from build123d import *

# Parameters (mm, degrees)
BOSS_EXTRUDE1_DEPTH     = 3
SKETCH2_W               = 33
SKETCH2_H               = 10
SKETCH2_R               = 1.25
BOSS_EXTRUDE2_DEPTH     = 3
SKETCH3_R               = 1.25
CUT_EXTRUDE1_DEPTH      = 111.114926801
BOSS_EXTRUDE3_DEPTH     = 10
CUT_EXTRUDE2_REACH      = 107.286
CUT_EXTRUDE2_END_RADIUS = 197.003812576
SKETCH8_R               = 1.5
CUT_EXTRUDE3_REACH      = 97.662
CUT_EXTRUDE3_END_RADIUS = 197.003812576
SKETCH9_R               = 1.5


with BuildPart() as part:
    # Sketch1 → Boss-Extrude1 (new body)
    with BuildSketch(Plane(origin=(0, 0, 0), x_dir=(1, 0, 0), z_dir=(0, 1, 0))):
        with BuildLine():
            Line((0, 45), (0, 0))
            Line((0, 0), (7, 0))
            Line((7, 0), (45.00148551, -17.720383715))
            Line((45.00148551, -17.720383715), (43.311012463, -21.345614863))
            Line((43.311012463, -21.345614863), (100.00148551, -17.720383715))
            Line((100.00148551, -17.720383715), (100.00148551, 12.279616285))
            ThreePointArc((100.00148551, 12.279616285), (52.191052923, 35.333931061), (0, 45))
        make_face()
    extrude(amount=BOSS_EXTRUDE1_DEPTH)

    # Sketch2 → Boss-Extrude2 (add)
    with BuildSketch(Plane(origin=(1.250243366, 0, -2.681155551), x_dir=(0.9063077870366495, 0, 0.42261826174070033), z_dir=(-0.42261826174070033, 0, 0.9063077870366495))):
        with Locations((22.844154509, 5)):
            Rectangle(SKETCH2_W, SKETCH2_H)
        with Locations((13.344154509, 6)):
            Circle(SKETCH2_R, mode=Mode.SUBTRACT)
        with Locations((32.344154509, 6)):
            Circle(SKETCH2_R, mode=Mode.SUBTRACT)
    extrude(amount=-BOSS_EXTRUDE2_DEPTH)

    # Sketch3 → Cut-Extrude1 (cut, through all)
    with BuildSketch(Plane.XZ):
        with Locations(Location((5, -23.5, 0), (0, 0, 270))):
            Circle(SKETCH3_R)
        with Locations(Location((92.00148551, 2.720383715, 0), (0, 0, 270))):
            Circle(SKETCH3_R)
    extrude(amount=-CUT_EXTRUDE1_DEPTH, mode=Mode.SUBTRACT)

    # Sketch6 → Boss-Extrude3 (add)
    with BuildSketch(Plane(origin=(0, 3, 0), x_dir=(1, 0, 0), z_dir=(0, 1, 0))):
        with BuildLine():
            ThreePointArc((25.815183319, 42.016667614), (17.915864182, 43.291962745), (9.971855225, 44.250264466))
            Line((9.971855225, 44.250264466), (9.971855225, 41.238788581))
            ThreePointArc((9.971855225, 41.238788581), (17.646509134, 40.304062324), (25.278576941, 39.068923955))
            Line((25.278576941, 39.068923955), (25.815183319, 42.016667614))
        make_face()
        with BuildLine():
            ThreePointArc((91.515126037, 17.56938971), (84.541117021, 21.492248202), (77.415775106, 25.13300679))
            Line((77.415775106, 25.13300679), (76.106143507, 22.438196193))
            ThreePointArc((76.106143507, 22.438196193), (83.124741123, 18.85197958), (89.994272948, 14.987889185))
            Line((89.994272948, 14.987889185), (91.515126037, 17.56938971))
        make_face()
    extrude(amount=BOSS_EXTRUDE3_DEPTH)

    # Cut-Extrude2: up to this cylinder (the profile starts outside it)
    cut_extrude2_end = Plane(origin=(-10.004096478, 8, 154.749638432), z_dir=(0, -1, 0)) * Cylinder(CUT_EXTRUDE2_END_RADIUS, 609.579625152, mode=Mode.PRIVATE)
    # Sketch8 → Cut-Extrude2 (cut, up to the surface)
    with BuildSketch(Plane(origin=(17.915864182, 13, -43.291962745), x_dir=(-0.9902080058846244, 0, -0.13959980330213892), z_dir=(0.13959980330213892, 0, -0.9902080058846244)), mode=Mode.PRIVATE) as cut_extrude2_sk1:
        with Locations((0, -5)):
            Circle(SKETCH8_R)
    cut_extrude2_tool1 = extrude(cut_extrude2_sk1.sketch, amount=-CUT_EXTRUDE2_REACH, mode=Mode.PRIVATE) - cut_extrude2_end
    add(cut_extrude2_tool1.solids().sort_by_distance((17.915864, 8, -43.291963))[0], mode=Mode.SUBTRACT)

    # Cut-Extrude3: up to this cylinder (the profile starts outside it)
    cut_extrude3_end = Plane(origin=(-10.004096478, 8, 154.749638432), z_dir=(0, -1, 0)) * Cylinder(CUT_EXTRUDE3_END_RADIUS, 590.331625152, mode=Mode.PRIVATE)
    # Sketch9 → Cut-Extrude3 (cut, up to the surface)
    with BuildSketch(Plane(origin=(84.541117021, 13, -21.492248202), x_dir=(-0.8812094331704029, 0, -0.4727260674973377), z_dir=(0.4727260674973377, 0, -0.8812094331704029)), mode=Mode.PRIVATE) as cut_extrude3_sk1:
        with Locations((0, -5)):
            Circle(SKETCH9_R)
    cut_extrude3_tool1 = extrude(cut_extrude3_sk1.sketch, amount=-CUT_EXTRUDE3_REACH, mode=Mode.PRIVATE) - cut_extrude3_end
    add(cut_extrude3_tool1.solids().sort_by_distance((84.541117, 8, -21.492248))[0], mode=Mode.SUBTRACT)


solid = part.part
Part model, mm, in its own coordinate system. A direction names the side the tool comes from. Coordinates: 2 decimals unless noted, no trailing zeros. Loops run counter-clockwise (first coordinate to the right, second up) from the corner with the lowest first, then second, coordinate; pieces in that order, holes last. Notation, with made-up numbers: (-6.75, 31) - (14.25, 31) arc R37 ccw to (14.25, 69) - close; hole circle Ø7 at (17.5, 65). An arc over 180 degrees is marked (long way). Write each question's results on one line, items separated by ' | '. Start each with the question number.
Q1. Which spindle directions (+Z, -Z, +X, -X, +Y, -Y) get a long thin tool onto all of the face, cutting with end or side? Do faces 5 (the flat face through (22, 10, 6)), 6 (the cylindrical face through (19.24, 7.93, -40.07)), 7 (the flat face through (7.625, 6.451, -1.34)), 8 (the flat face through (90.744, 7.93, -16.261)), 9 (the cylindrical face through (81.48, 7.93, -19.724)). Say none if no direction does.
Q2. Two-plate mould, pull along Y, no slides. Class faces 1 (the cylindrical face through (13.72, 4.78, 1.5)), 2 (the flat face through (0, 1, -23)), 3 (the flat face through (49, 0, -12)), 4 (the flat face through (84, 13, -20)): +Y half, -Y half, draft (parallel to the pull), parting line (faces both ways), or undercut.
Q3. Slice it at B-B on x = 5. Give the cut face in (y, z), and give its area (3 significant figures).
Q4. Slice it at A-A on z = -23.5. Give the cut face in (x, y).
Q5. Drop flat-ended pins along their axis: pin 1 Ø8.5 at (x, z) = (25, 7) entering from +Y; pin 2 Ø2.5 at (x, y) = (4, 1) entering from +Z; pin 3 Ø3 at (x, y) = (83.5, 8) entering from +Z. Give the stop position or say it passes through.
Q6. Probe line 1 along Y through (x, z) = (61.5, -17.5); line 2 along Z through (x, y) = (12.5, 3.75); line 3 along X through (y, z) = (1.55, -23.5). List the from-to ranges inside material, lowest first.
Q7. Slice it at C-C on y = 1. Give the cut face in (x, z), and give its area (3 significant figures).
Q8. Slice it at D-D on x = 68.5. Give the cut face in (y, z).
Answer:
1) face 5: +Z, +X, -X, +Y | face 6: -X, +Y | face 7: -Z, -X, +Y | face 8: +Z, +X, +Y | face 9: +Z, -X, +Y
2) face 1: undercut | face 2: draft | face 3: -Y half | face 4: +Y half
3) outline: (0, -44.69) - (3, -44.69) - (3, -24.75) - (0, -24.75) - close; (0, -22.25) - (3, -22.25) - (3, 0) - (0, 0) - close | area: 127 mm2
4) outline: (0, 0) - (3.75, 0) - (3.75, 3) - (0, 3) - close; (6.25, 0) - (80.7, 0) - (80.7, 13) - (76.62, 13) - (76.62, 3) - (6.25, 3) - close
5) pin 1: stops at y = 10 | pin 2: stops at z = 0 | pin 3: stops at z = -17.83
6) line 1: y = 0 to 3 | line 2: z = -43.98 to -40.96, -0.75 to 2.56 | line 3: x = 0 to 3.75, 6.25 to 80.7
7) outline: (0, -45) arc R200 ccw to (100, -12.28) - (100, 17.72) - (43.31, 21.35) - (45, 17.72) - (7, 0) - (0, 0) - close; hole circle Ø2.5 at (5, -23.5); hole circle Ø2.5 at (92, 2.72) | area: 4,760 mm2
8) outline: (0, -29.2) - (3, -29.2) - (3, 19.73) - (0, 19.73) - close
